Design review of the part shown in the three views and the two pictorial views. Dimensions are in mm from the part's minimum x, y and z. A direction names the side the tool comes from. Coordinates: 2 decimals unless noted, no trailing zeros. Write each loop counter-clockwise with the first axis right and the second up, starting at its lowest first coordinate (ties: lowest second). Pieces come first, ordered by that corner, then holes. Notation, with made-up numbers: M -18,75.5 L 2,75.5 A24 ccw 2,95.5 Z; hole C -11.5,-34 d4. An arc over 180 degrees is marked long. One line per question, with ' | ' between items.
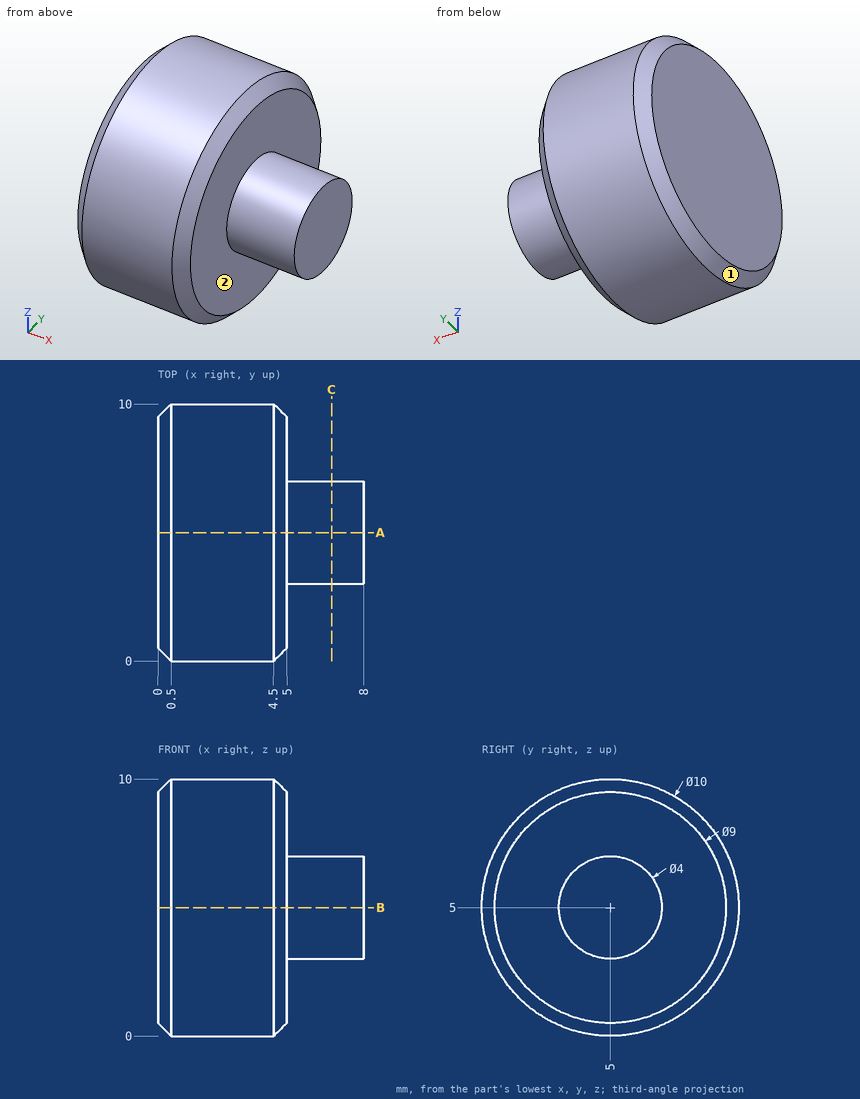
1. For line 1 along X through (y, z) = (4, 8.25); line 2 along X through (y, z) = (2.25, 1.25); line 3 along Z through (x, y) = (3.5, 9.5), list the stretches that pass through material, from the lowest coordinate up.
Computed values:
line 1: x = 0 to 5 | line 2: x = 0.15 to 4.85 | line 3: z = 2.82 to 7.18
2. Machinability: for the marked faces 1 and 2, which of the approach directions +Z, -Z, +X, -X, +Y, -Y give a long, thin tool a straight path to every point of the face, cutting with its end or side? Answer none if there is none.
Computed values:
face 1: -X | face 2: +X
3. Take a section at C-C on x = 6.75. State the section outline as (y, z) points, plus the area to 3 significant figures.
Computed values:
outline: C 5,5 d4 | area: 12.6 mm2
4. Take a section at A-A on y = 5. State the section outline as (x, z) points, plus the area to 3 significant figures.
Computed values:
outline: M 0,0.5 L 0.5,0 L 4.5,0 L 5,0.5 L 5,3 L 8,3 L 8,7 L 5,7 L 5,9.5 L 4.5,10 L 0.5,10 L 0,9.5 Z | area: 61.5 mm2
5. Clearance check with flat-ended pins moving along their axes: P1, Ø2, axis at x = 1, y = 1.5, coming from the -Z side; P2, Ø1, axis at x = 1.5, y = 5.5, coming from the -Z side; P3, Ø1, axis at y = 4.5, z = 1.5, coming from the +X side. State where each tip first meets the part, or that it passes through.
Computed values:
P1: stops at z = 0.67 | P2: stops at z = 0 | P3: stops at x = 5
